Part print with two shaded views. Sizes in mm from the minimum x, y, z corner. Coordinates: 2 decimals unless noted, no trailing zeros. Loops run counter-clockwise (first coordinate to the right, second up) from the corner with the lowest first, then second, coordinate; pieces in that order, holes last.
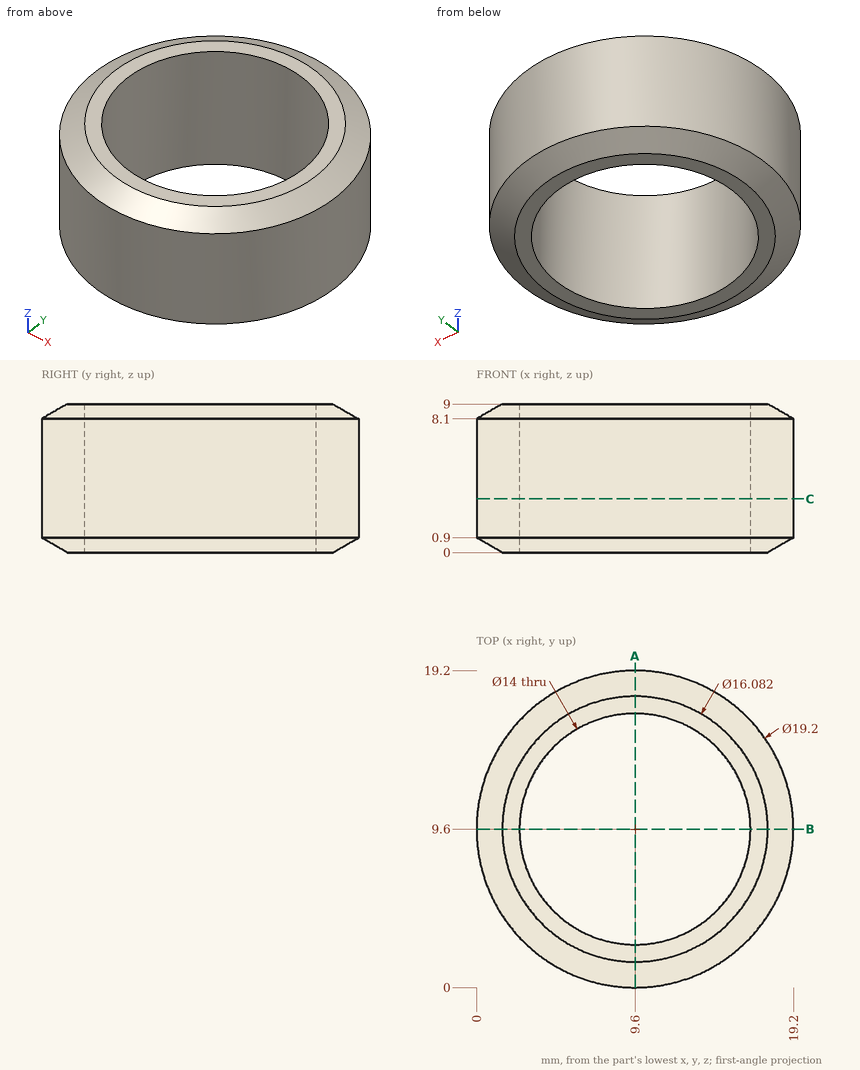
Q1. Slice it at A-A (x = 9.6). List the corners of the cut face in (y, z), and give its area (3 significant figures).
Answers:
outline: (0, 0.9) - (1.56, 0) - (2.6, 0) - (2.6, 9) - (1.56, 9) - (0, 8.1) - close; (16.6, 0) - (17.64, 0) - (19.2, 0.9) - (19.2, 8.1) - (17.64, 9) - (16.6, 9) - close
area: 44.0 mm2
Q2. Drill centre lines: line 1 (Y direction, x = 9.6, z = 7.25); line 2 (Y direction, x = 13.75, z = 1.5); line 3 (X direction, y = 10.75, z = 4) (1 decimal). Where is each one in solid material? Low to high.
Answers:
line 1: y = 0 to 2.6, 16.6 to 19.2
line 2: y = 0.94 to 3.96, 15.24 to 18.26
line 3: x = 0.1 to 2.7, 16.5 to 19.1
Q3. Flat gauge pins, fed straight in: P1, Ø5, axis at y = 13, z = 6, coming from the +X side; P2, Ø3, axis at y = 5.5, z = 2, coming from the -X side; P3, Ø4, axis at x = 7, z = 3, coming from the +Y side. Where does each tip first touch, or does it go through?
Answers:
P1: stops at x = 19.16
P2: stops at x = 0.36
P3: stops at y = 19.18
Q4. Slice it at C-C (z = 3.25). List the corners of the cut face in (x, y).
Answers:
outline: circle Ø19.2 at (9.6, 9.6); hole circle Ø14 at (9.6, 9.6)
